Part model, mm, in its own coordinate system. Give positions to 0.01 mm unless a question says otherwise; leave off trailing zeros. Order: outer loops, then holes, each group sorted by start corner. A loop starts at its lowest first (then second) coordinate and runs counter-clockwise, first axis right, second up.
1. Drop flat-ended pins along their axis: pin 1 Ø17.5 at (x, z) = (31, -16) entering from +Y; pin 2 Ø1 at (y, z) = (1.5, -31) entering from +X; pin 3 Ø0.6 at (y, z) = (3, -8) entering from +X. Give the stop position or say it passes through.
2. Slice it at C-C on y = 1.7. Give the number of separate pieces and of enclosed holes in the cut face, and give its area (3 significant figures).
3. Mould opens along Z. For faces 1 (the cylindrical face through (123.01, 1.22, -8.27)), 2 (the flat face through (118, 2.4, -22)), 3 (the cylindrical face through (-61.4, 1.217, -34.485)), 4 (the cylindrical face through (-44.683, 1.217, -24.372)) say: +Z half, -Z half, draft (parallel to the pull), parting line (faces both ways), or undercut.
4. Slice it at B-B on x = 4. List the corners of the cut face in (y, z), and give its area (3 significant figures).
5. Probe line 1 (Z direction, x = 105.5, y = 1.65); line 2 (X direction, y = 0.7, z = -23); line 3 (X direction, y = 2.2, z = -15). List the from-to ranges inside material, lowest first.
6. Slice it at A-A on x = 107.5. List the corners of the cut face in (y, z), and give its area (3 significant figures).
from build123d import *

# Parameters (mm, degrees)
SKETCH1_W           = 193.2
SKETCH1_H           = 35
BOSS_EXTRUDE1_DEPTH = 2.4
SKETCH2_R           = 1.13
SKETCH2_R_2         = 3.625
SKETCH2_R_3         = 0.5
SKETCH2_W           = 40
SKETCH2_H           = 20
CUT_EXTRUDE1_DEPTH  = 2.4
SKETCH4_W           = 4
SKETCH4_H           = 6
CUT_EXTRUDE2_DEPTH  = 2.4
FILLET1_R           = 15
FILLET2_R           = 2
SKETCH5_W           = 0.5
SKETCH5_H           = 7.5
BOSS_EXTRUDE2_DEPTH = 0.5


with BuildPart() as part:
    # Sketch1 → Boss-Extrude1 (new body)
    with BuildSketch(Plane(origin=(0, 0, 0), x_dir=(1, 0, 0), z_dir=(0, 1, 0))):
        with Locations((30.922946176, 21.495750708)):
            Rectangle(SKETCH1_W, SKETCH1_H)
    extrude(amount=BOSS_EXTRUDE1_DEPTH)

    # Sketch2 → Cut-Extrude1 (cut)
    with BuildSketch(Plane(origin=(0, 2.4, 0), x_dir=(1, 0, 0), z_dir=(0, 1, 0))):
        with Locations(Location((66.522946176, 26.495750708, 0), (0, 0, 270))):
            Circle(SKETCH2_R)
        with Locations(Location((118.522946176, 26.495750708, 0), (0, 0, 270))):
            Circle(SKETCH2_R)
        with Locations(Location((118.522946176, 16.495750708, 0), (0, 0, 90))):
            Circle(SKETCH2_R)
        with Locations(Location((66.522946176, 16.495750708, 0), (0, 0, 90))):
            Circle(SKETCH2_R)
        with Locations(Location((-42.477053824, 21.495750708, 0), (0, 0, 270))):
            Circle(SKETCH2_R_2)
        with Locations(Location((-49.907053824, 21.495750708, 0), (0, 0, 270))):
            Circle(SKETCH2_R_3)
        with Locations(Location((-52.842053824, 21.495750708, 0), (0, 0, 270))):
            Circle(SKETCH2_R_3)
        with Locations(Location((-55.847053824, 21.495750708, 0), (0, 0, 270))):
            Circle(SKETCH2_R_3)
        with Locations(Location((-49.162053824, 33.074510357, 0), (0, 0, 270))):
            Circle(SKETCH2_R_3)
        with Locations(Location((-47.659553824, 30.472104018, 0), (0, 0, 270))):
            Circle(SKETCH2_R_3)
        with Locations(Location((-46.192053824, 27.930319458, 0), (0, 0, 270))):
            Circle(SKETCH2_R_3)
        with Locations(Location((-35.792053824, 33.074510357, 0), (0, 0, 270))):
            Circle(SKETCH2_R_3)
        with Locations(Location((-37.294553824, 30.472104018, 0), (0, 0, 270))):
            Circle(SKETCH2_R_3)
        with Locations(Location((-38.762053824, 27.930319458, 0), (0, 0, 270))):
            Circle(SKETCH2_R_3)
        with Locations(Location((-29.107053824, 21.495750708, 0), (0, 0, 270))):
            Circle(SKETCH2_R_3)
        with Locations(Location((-32.112053824, 21.495750708, 0), (0, 0, 270))):
            Circle(SKETCH2_R_3)
        with Locations(Location((-35.047053824, 21.495750708, 0), (0, 0, 270))):
            Circle(SKETCH2_R_3)
        with Locations(Location((-35.792053824, 9.91699106, 0), (0, 0, 270))):
            Circle(SKETCH2_R_3)
        with Locations(Location((-37.294553824, 12.519397398, 0), (0, 0, 270))):
            Circle(SKETCH2_R_3)
        with Locations(Location((-38.762053824, 15.061181958, 0), (0, 0, 270))):
            Circle(SKETCH2_R_3)
        with Locations(Location((-49.162053824, 9.91699106, 0), (0, 0, 270))):
            Circle(SKETCH2_R_3)
        with Locations(Location((-47.659553824, 12.519397398, 0), (0, 0, 270))):
            Circle(SKETCH2_R_3)
        with Locations(Location((-46.192053824, 15.061181958, 0), (0, 0, 270))):
            Circle(SKETCH2_R_3)
        with Locations((92.522946176, 21.495750708)):
            Rectangle(SKETCH2_W, SKETCH2_H)
    extrude(amount=-CUT_EXTRUDE1_DEPTH, mode=Mode.SUBTRACT)

    # Sketch4 → Cut-Extrude2 (cut)
    with BuildSketch(Plane(origin=(0, 2.4, 0), x_dir=(1, 0, 0), z_dir=(0, 1, 0))):
        with Locations((114.522946176, 21.495750708)):
            Rectangle(SKETCH4_W, SKETCH4_H)
    extrude(amount=-CUT_EXTRUDE2_DEPTH, mode=Mode.SUBTRACT)

    # Fillet1
    fillet1_edges = [part.edges().sort_by_distance(p)[0] for p in [
        (-65.677053824, 1.2, -38.995750708),
        (127.522946176, 1.2, -38.995750708),
        (127.522946176, 1.2, -3.995750708),
        (-65.677053824, 1.2, -3.995750708),
    ]]
    fillet(fillet1_edges, radius=FILLET1_R)

    # Fillet2
    fillet2_edges = [part.edges().sort_by_distance(p)[0] for p in [
        (112.522946176, 1.2, -18.495750708),
        (112.522946176, 1.2, -24.495750708),
    ]]
    fillet(fillet2_edges, radius=FILLET2_R)

    # Sketch5 → Boss-Extrude2 (add)
    with BuildSketch(Plane(origin=(0, 2.4, 0), x_dir=(1, 0, 0), z_dir=(0, 1, 0))):
        with Locations((102.522946176, 35.245750708)):
            Rectangle(SKETCH5_W, SKETCH5_H)
        with Locations((102.522946176, 7.745750708)):
            Rectangle(SKETCH5_W, SKETCH5_H)
        with Locations((-42.477053824, 7.745750708)):
            Rectangle(SKETCH5_W, SKETCH5_H)
        with Locations((-42.477053824, 35.245750708)):
            Rectangle(SKETCH5_W, SKETCH5_H)
    extrude(amount=BOSS_EXTRUDE2_DEPTH)


solid = part.part
Data:
1. pin 1: stops at y = 2.4
1. pin 2: stops at x = 126.04
1. pin 3: stops at x = 102.77
2. separate pieces: 1
2. enclosed holes: 24
2. area: 5,670 mm2
3. face 1: +Z half
3. face 2: draft
3. face 3: -Z half
3. face 4: undercut
4. outline: (0, -39) - (2.4, -39) - (2.4, -4) - (0, -4) - close
4. area: 84.0 mm2
5. line 1: z = -39 to -31.5, -11.5 to -4
5. line 2: x = -65.68 to -45.78, -39.18 to 72.52, 116.52 to 127.52
5. line 3: x = -65.14 to -46.69, -45.7 to -39.26, -38.27 to 72.52, 112.52 to 126.98
6. outline: (0, -39) - (2.4, -39) - (2.4, -31.5) - (0, -31.5) - close; (0, -11.5) - (2.4, -11.5) - (2.4, -4) - (0, -4) - close
6. area: 36.0 mm2
